Input: dimensioned drawing with shaded views. Units: mm. Origin: part minimum x, y, z. Give positions to 0.01 mm unless a question says otherwise; leave off trailing zeros. Order: outer loops, then holes, each group sorted by start corner. A loop starts at its lowest first (then second) coordinate and runs counter-clockwise, first axis right, second up. Notation, with made-up numbers: M -25.75,-26.75 L -17.75,-26.75 A24 cw -17.75,3.25 Z; hole C -9.75,78 d11. An arc over 180 degrees is marked long. Answer in a Markdown table with one row per item. Add a question column.
(1) Mould query, pull axis X, two halves, no side actions, for the marked faces 1 and 2. Classes: pulls with the +X half, pulls with the -X half, needs draft (parallel to the pull), parting line crosses it, or undercut.
(2) Section query A-A, the plane z = 2.1. Return loops of the section in (x, y).
(3) Material intervals for line 1 along X through (y, z) = (1.25, 1.5); line 2 along Z through (x, y) = (14, 0.5); line 3 along Y through (x, z) = (27, 0.3), sorted ascending.
(4) Section query C-C, the plane x = 14.5. Return loops of the section in (y, z), plus the area to 3 significant figures.
(5) Pin query (flat end, axial travel): P1, Ø1, axis at y = 3.5, z = 2, coming from the +X side; P2, Ø0.8, axis at x = 21.5, y = 0.5, coming from the +Z side; P3, Ø0.8, axis at y = 3.5, z = 1.5, coming from the -X side. Return the tip coordinate at first contact, or that it passes through.
(6) Section query B-B, the plane y = 2. Return loops of the section in (x, z).
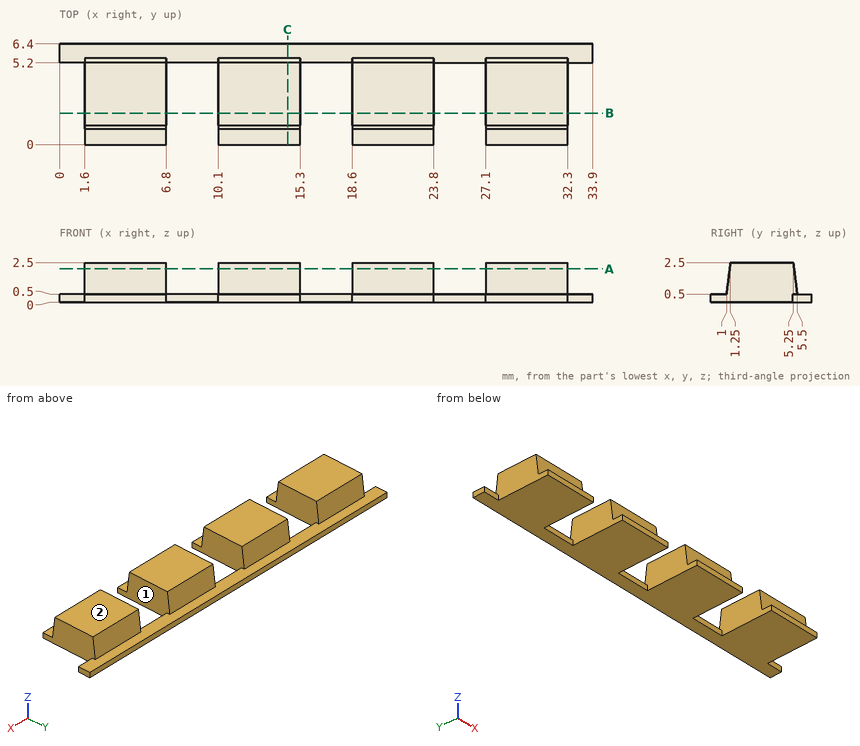
Values follow:
| question | item | result |
|---|---|---|
| 1 | face 1 | undercut |
| 1 | face 2 | needs draft |
| 2 | outline | M 1.6,1.2 L 6.8,1.2 L 6.8,5.3 L 1.6,5.3 Z; M 10.1,1.2 L 15.3,1.2 L 15.3,5.3 L 10.1,5.3 Z; M 18.6,1.2 L 23.8,1.2 L 23.8,5.3 L 18.6,5.3 Z; M 27.1,1.2 L 32.3,1.2 L 32.3,5.3 L 27.1,5.3 Z |
| 3 | line 1 | x = 1.6 to 6.8, 10.1 to 15.3, 18.6 to 23.8, 27.1 to 32.3 |
| 3 | line 2 | z = 0 to 0.5 |
| 3 | line 3 | y = 5.2 to 6.4 |
| 4 | outline | M 0,0 L 6.4,0 L 6.4,0.5 L 5.5,0.5 L 5.25,2.5 L 1.25,2.5 L 1,0.5 L 0,0.5 Z |
| 4 | area | 11.7 mm² |
| 5 | P1 | stops at x = 32.3 |
| 5 | P2 | stops at z = 0.5 |
| 5 | P3 | stops at x = 1.6 |
| 6 | outline | M 1.6,0 L 6.8,0 L 6.8,2.5 L 1.6,2.5 Z; M 10.1,0 L 15.3,0 L 15.3,2.5 L 10.1,2.5 Z; M 18.6,0 L 23.8,0 L 23.8,2.5 L 18.6,2.5 Z; M 27.1,0 L 32.3,0 L 32.3,2.5 L 27.1,2.5 Z |
